Design review of the part built by this model. Coordinates are the model's own, in mm. Face numbers are marked on the shaded views. A direction names the side the tool comes from. Coordinates: 2 decimals unless noted, no trailing zeros. Write each loop counter-clockwise with the first axis right and the second up, starting at its lowest first coordinate (ties: lowest second). Pieces come first, ordered by that corner, then holes.
Q1. Add section D-D, the plane x = 11. Give the boundary of the cut face in (y, z), plus the area to 3 significant figures.
Q2. Machinability: for the marked faces 4 and 5, which of the approach directions +Z, -Z, +X, -X, +Y, -Y give a long, thin tool a straight path to every point of the face, cutting with its end or side? Answer none if there is none.
Q3. Add section B-B, the plane y = 0. Give the boundary of the cut face in (x, z), plus the area to 3 significant figures.
Q4. Clearance check with flat-ended pins moving along their axes: pin 1 Ø5 at (x, y) = (0, 11.5) entering from -Z; pin 2 Ø2 at (y, z) = (-6.5, -2) entering from -X; pin 3 Ø3 at (y, z) = (-6.5, 5) entering from +X. State where each tip first meets the part, or that it passes through.
Q5. To check wall thickness, follow probe 1 along X at (y, z) = (-5, 1); probe 2 along Y at (x, z) = (0, 0.8); probe 3 along Y at (x, z) = (0, 13). State the ranges of each line that lie inside material, in increasing order.
Q6. Add section C-C, the plane z = 12.5. Give the boundary of the cut face in (x, y), plus the area to 3 significant figures.
Q7. The part is to be moulded in two halves that separate along Y. For the marked faces 1, 2 and 3, say which applies: +Y half, -Y half, draft (parallel to the pull), parting line (faces both ways), or undercut.
Q8. Add section A-A, the plane x = 0. Give the boundary of the cut face in (y, z), plus the area to 3 significant figures.
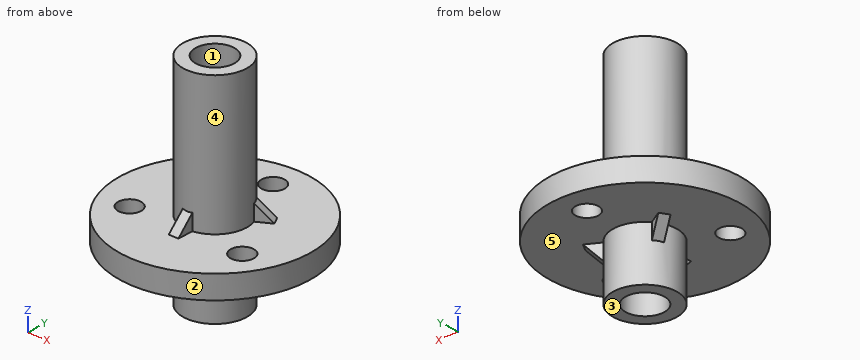
from build123d import *

# Parameters (mm, degrees)
CROQUIS1_R              = 16.5
CROQUIS1_R_2            = 2
SALIENTE_EXTRUIR1_DEPTH = 4
CROQUIS2_R              = 5.5
SALIENTE_EXTRUIR2_DEPTH = 23.8
SALIENTE_EXTRUIR3_START = 9.4
CROQUIS3_R              = 5.5
SALIENTE_EXTRUIR3_DEPTH = 9.4
CROQUIS5_R              = 3.35
CORTAR_EXTRUIR1_DEPTH   = 37.2
SALIENTE_EXTRUIR7_DEPTH = 0.85
MATRIZC1_COUNT          = 3
SIMETR_A1_COPY_1_DEPTH  = 0.85
SIMETR_A1_COPY_2_DEPTH  = 0.85


with BuildPart() as part:
    # Croquis1 → Saliente-Extruir1 (new body)
    with BuildSketch(Plane.XY):
        Circle(CROQUIS1_R)
        with Locations((0, 11.5)):
            Circle(CROQUIS1_R_2, mode=Mode.SUBTRACT)
        with Locations((-9.959292144, -5.75)):
            Circle(CROQUIS1_R_2, mode=Mode.SUBTRACT)
        with Locations((9.959292144, -5.75)):
            Circle(CROQUIS1_R_2, mode=Mode.SUBTRACT)
    extrude(amount=SALIENTE_EXTRUIR1_DEPTH)

    # Croquis2 → Saliente-Extruir2 (add)
    with BuildSketch(Plane.XY.offset(4)):
        Circle(CROQUIS2_R)
    extrude(amount=SALIENTE_EXTRUIR2_DEPTH)

    # Croquis3 → Saliente-Extruir3 (add)
    with BuildSketch(Plane(origin=(0, 0, 0), x_dir=(-1, 0, 0), z_dir=(0, 0, -1)).offset(SALIENTE_EXTRUIR3_START)):
        with Locations(Location((0, 0, 0), (0, 0, 180))):
            Circle(CROQUIS3_R)
    extrude(amount=-SALIENTE_EXTRUIR3_DEPTH)

    # Croquis5 → Cortar-Extruir1 (cut)
    with BuildSketch(Plane.XY.offset(27.8)):
        Circle(CROQUIS5_R)
    extrude(amount=-CORTAR_EXTRUIR1_DEPTH, mode=Mode.SUBTRACT)

    # Croquis7 → Saliente-Extruir7 (add, symmetric)
    with BuildSketch(Plane(origin=(0, 0, 0), x_dir=(0, 0, -1), z_dir=(1, 0, 0))):
        Polygon((-4, -4.874650825), (-4, -5.5), (-6.7, -5.5), (-7.325349175, -4.874650825), align=None)
        Polygon((-6.7, -5.5), (-4, -8.2), (-4, -5.5), align=None)
    saliente_extruir7 = extrude(amount=SALIENTE_EXTRUIR7_DEPTH, both=True)

    # MatrizC1: Saliente-Extruir7 ×3 about axis
    matrizc1_axis = Axis((0, 0, -18.875230868), (0, 0, 1))
    for i in range(1, MATRIZC1_COUNT):
        add(saliente_extruir7.rotate(matrizc1_axis, i * 360 / MATRIZC1_COUNT))

    # Simetría1: Saliente-Extruir7 across plane
    add(saliente_extruir7.mirror(Plane.XY.offset(2)))

    # Simetría1 copy 1 sketch → Simetría1 copy 1 (add, symmetric)
    with BuildSketch(Plane(origin=(0, 0, 4), x_dir=(0, 0, 1), z_dir=(-0.4999999999999998, 0.8660254037844387, 0))):
        Polygon((-4, 4.874650825), (-4, 5.5), (-6.7, 5.5), (-7.325349175, 4.874650825), align=None)
        Polygon((-6.7, 5.5), (-4, 8.2), (-4, 5.5), align=None)
    extrude(amount=SIMETR_A1_COPY_1_DEPTH, both=True)

    # Simetría1 copy 2 sketch → Simetría1 copy 2 (add, symmetric)
    with BuildSketch(Plane(origin=(0, 0, 4), x_dir=(0, 0, 1), z_dir=(-0.5000000000000004, -0.8660254037844384, 0))):
        Polygon((-4, 4.874650825), (-4, 5.5), (-6.7, 5.5), (-7.325349175, 4.874650825), align=None)
        Polygon((-6.7, 5.5), (-4, 8.2), (-4, 5.5), align=None)
    extrude(amount=SIMETR_A1_COPY_2_DEPTH, both=True)


solid = part.part
Here are the results:
1. outline: (-12.3, 0) - (-7.46, 0) - (-7.46, 4) - (-12.3, 4) - close; (-4.04, 0) - (12.3, 0) - (12.3, 4) - (-4.04, 4) - close
1. area: 84.7 mm2
2. face 4: +Z
2. face 5: -Z
3. outline: (-16.5, 0) - (-5.5, 0) - (-5.5, -9.4) - (-3.35, -9.4) - (-3.35, 27.8) - (-5.5, 27.8) - (-5.5, 4) - (-16.5, 4) - close; (3.35, -9.4) - (5.5, -9.4) - (5.5, 0) - (16.5, 0) - (16.5, 4) - (5.5, 4) - (5.5, 27.8) - (3.35, 27.8) - close
3. area: 248 mm2
4. pin 1: stops at z = 0
4. pin 2: stops at x = -0.85
4. pin 3: stops at x = 15.6
5. probe 1: x = -15.72 to -11.81, -8.11 to 8.11, 11.81 to 15.72
5. probe 2: y = -16.5 to -3.35, 3.35 to 9.5, 13.5 to 16.5
5. probe 3: y = -5.5 to -3.35, 3.35 to 5.5
6. outline: circle Ø11 at (0, 0); hole circle Ø6.7 at (0, 0)
6. area: 59.8 mm2
7. face 1: undercut
7. face 2: parting line
7. face 3: draft
8. outline: (-16.5, 0) - (-8.2, 0) - (-5.5, -2.7) - (-5.5, -9.4) - (-3.35, -9.4) - (-3.35, 27.8) - (-5.5, 27.8) - (-5.5, 6.7) - (-8.2, 4) - (-16.5, 4) - close; (3.35, -9.4) - (5.5, -9.4) - (5.5, 0) - (9.5, 0) - (9.5, 4) - (5.5, 4) - (5.5, 27.8) - (3.35, 27.8) - close; (13.5, 0) - (16.5, 0) - (16.5, 4) - (13.5, 4) - close
8. area: 239 mm2
